Source: three-view drawing plus pictorial views. Frame: mm from the lowest corner of the part. Round coordinates to 2 decimals unless told otherwise and drop trailing zeros. Loops run counter-clockwise (first coordinate to the right, second up) from the corner with the lowest first, then second, coordinate; pieces in that order, holes last. Notation, with made-up numbers: (-39.5, 64) -> (-26.5, 64) arc R18 ccw to (-26.5, 81) -> close; hole circle Ø7 at (-3.5, 83). An arc over 180 degrees is marked (long way). Answer in a Markdown table with one row per item. Add a question column.
Q1. Section A-A, the plane x = 83.5. Output: boundary loops of the cut face in (y, z), and give its area (3 significant figures).
Q2. Pin query (flat end, axial travel): pin 1 (1 mm diameter, centred on x = 79, z = 11.5, fed in from +Y); pin 2 (1.5 mm diameter, centred on x = 63.5, y = 33, fed in from +Z) (1 decimal); pin 3 (10 mm diameter, centred on x = 45, z = 23, fed in from +Y). Return the tip coordinate at first contact, or that it passes through.
Q3. Ray query, L1, parallel to Z at x = 9.5, y = 36; L2, parallel to Z at x = 20, y = 41.5; L3, parallel to Y at x = 76, z = 24.5. Return the intervals inside material, ascending. Write a range as from..to.
Q4. Section B-B, the plane z = 25. Output: boundary loops of the cut face in (x, y), and give its area (3 significant figures).
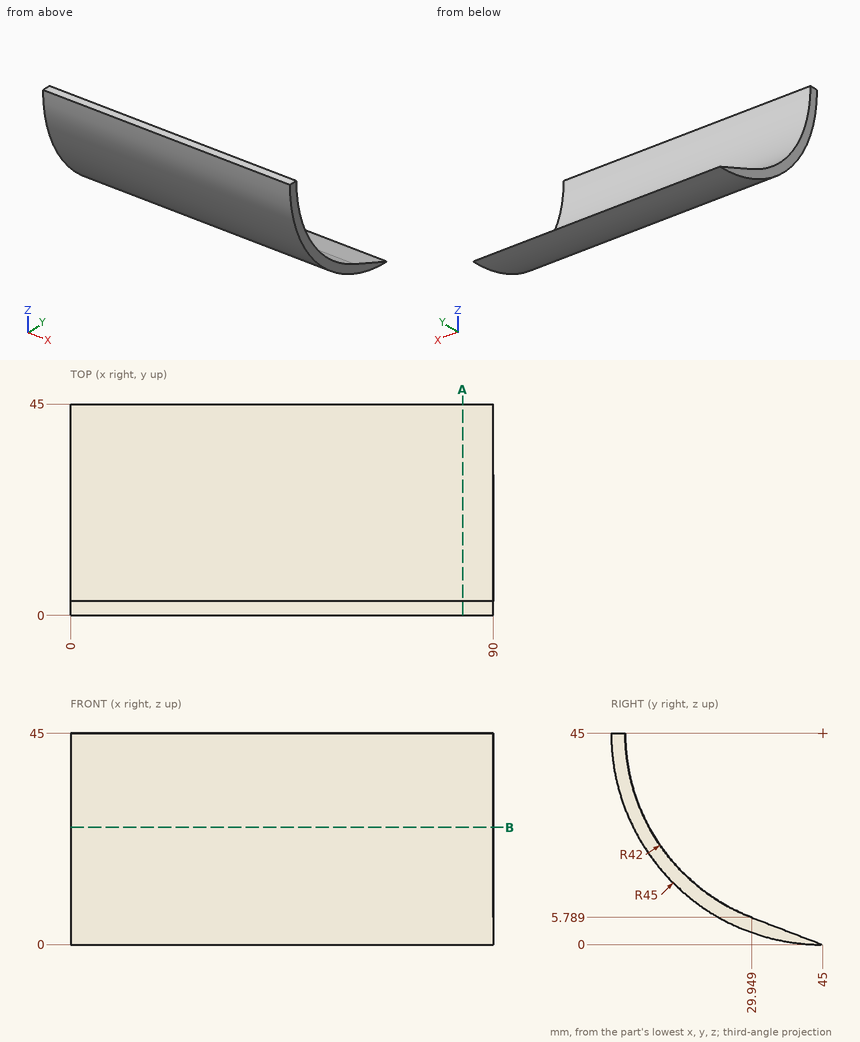
Answer block:
| question | item | result |
|---|---|---|
| 1 | outline | (0, 45) arc R45 ccw to (45, 0) -> (29.95, 5.79) arc R42 cw to (3, 45) -> close |
| 1 | area | 190 mm^2 |
| 2 | pin 1 | y = 20.34 |
| 2 | pin 2 | z = 4.9 |
| 2 | pin 3 | y = 12.83 |
| 3 | L1 | 0.91..3.46 |
| 3 | L2 | 0.14..1.35 |
| 3 | L3 | 4.94..8.34 |
| 4 | outline | (0, 4.69) -> (90, 4.69) -> (90, 8.07) -> (0, 8.07) -> close |
| 4 | area | 304 mm^2 |
